from build123d import *

# Parameters (mm, degrees)
F1_DEPTH = 20


with BuildPart() as f1:
    # F0 (on Top) → F1 (new body)
    with BuildSketch(Plane.XY):
        with BuildLine():
            Line((-4.08337, 18.350895), (0, 18.350895))
            Line((0, 18.350895), (4.08337, 18.350895))
            ThreePointArc((4.08337, 18.350895), (8.797416, 19.531724), (12.398165, 22.795339))
            ThreePointArc((12.398165, 22.795339), (25.178356, 23.493196), (22.271844, 11.028346))
            ThreePointArc((22.271844, 11.028346), (18.432547, 8.049022), (16.451072, 3.611642))
            Line((16.451072, 3.611642), (12.878556, -16.649105))
            ThreePointArc((12.878556, -16.649105), (14.054737, -18.328866), (15.734498, -17.152685))
            Line((15.734498, -17.152685), (19.307015, 3.108062))
            ThreePointArc((19.307015, 3.108062), (20.713862, 6.258602), (23.439763, 8.373922))
            ThreePointArc((23.439763, 8.373922), (27.399884, 25.35728), (9.986874, 24.40645))
            ThreePointArc((9.986874, 24.40645), (7.430343, 22.089283), (4.08337, 21.250895))
            Line((4.08337, 21.250895), (0, 21.250895))
            Line((0, 21.250895), (-4.08337, 21.250895))
            ThreePointArc((-4.08337, 21.250895), (-7.430343, 22.089283), (-9.986874, 24.40645))
            ThreePointArc((-9.986874, 24.40645), (-27.399884, 25.35728), (-23.439763, 8.373922))
            ThreePointArc((-23.439763, 8.373922), (-20.713862, 6.258602), (-19.307015, 3.108062))
            Line((-19.307015, 3.108062), (-15.734498, -17.152685))
            ThreePointArc((-15.734498, -17.152685), (-14.054737, -18.328866), (-12.878556, -16.649105))
            Line((-12.878556, -16.649105), (-16.451072, 3.611642))
            ThreePointArc((-16.451072, 3.611642), (-18.432547, 8.049022), (-22.271844, 11.028346))
            ThreePointArc((-22.271844, 11.028346), (-25.178356, 23.493196), (-12.398165, 22.795339))
            ThreePointArc((-12.398165, 22.795339), (-8.797416, 19.531724), (-4.08337, 18.350895))
        make_face()
    extrude(amount=F1_DEPTH)


solid = f1.part
Build history of the part. All positions in model axes, mm. A direction names the side the tool comes from. Coordinates: 2 decimals unless noted, no trailing zeros. Order: outer loops, then holes, each group sorted by start corner. A loop starts at its lowest first (then second) coordinate and runs counter-clockwise, first axis right, second up. Notation, with made-up numbers: (-38, 72.25) - (-18, 72.25) arc R11 ccw to (-18, 91.25) - close; hole circle Ø9 at (63, -13). An arc over 180 degrees is marked (long way). Write each question's results on one line, items separated by ' | '. Start each with the question number.
Item 1: Band-saw the part on D-D on y = 7.5. Write the cut outline in (x, z).
Item 2: Band-saw the part on A-A on y = 23.5. Write the cut outline in (x, z), and give its area (3 significant figures).
Item 3: Band-saw the part on B-B on x = 26. Write the cut outline in (y, z), and give its area (3 significant figures).
Item 4: Tool access for faces 1 (the face through (-17.546, -6.88, 9.86)), 2 (the face through (0, 18.351, 10)), 3 (the face through (0, 21.251, 10)), 4 (the face through (-18.39, 7.995, 9.86)): list every direction of +Z, -Z, +X, -X, +Y, -Y with a clear straight run to the whole face (end or side of a thin tool).
Item 5: Flat gauge pins, fed straight in: pin 1 (6 mm diameter, centred on y = 7, z = 4.5, fed in from -X); pin 2 (2.5 mm diameter, centred on x = -1.5, z = 6.5, fed in from +Y); pin 3 (1 mm diameter, centred on x = 7, z = 10.5, fed in from +Y). Where does each tip first touch, or does it go through?
Item 6: Band-saw the part on C-C on z = 19. Write the cut outline in (x, y), and give its area (3 significant figures).
Item 7: Mould opens along X. For faces 5 (the face through (0, 20, 0)), 6 (the face through (-20.744, 6.297, 9.86)), 7 (the face through (20.684, 6.22, 9.86)), 8 (the face through (14.023, -18.323, 9.86)) say: released by +X, released by -X, zero draft, split by the parting line, or undercut.
Item 8: Wall check: probe 1 along X at (y, z) = (24, 19); probe 2 along Y at (x, z) = (-0.5, 14); probe 3 along X at (y, z) = (25, 11.75). Give the ranges that are in metal, low to high. Write a range as [from, to].
Numbers:
1) outline: (-21.97, 0) - (-18.03, 0) - (-18.03, 20) - (-21.97, 20) - close; (18.03, 0) - (21.97, 0) - (21.97, 20) - (18.03, 20) - close
2) outline: (-28.66, 0) - (-25.17, 0) - (-25.17, 20) - (-28.66, 20) - close; (-12.93, 0) - (-9.27, 0) - (-9.27, 20) - (-12.93, 20) - close; (9.27, 0) - (12.93, 0) - (12.93, 20) - (9.27, 20) - close; (25.17, 0) - (28.66, 0) - (28.66, 20) - (25.17, 20) - close | area: 286 mm^2
3) outline: (9.95, 0) - (14.39, 0) - (14.39, 20) - (9.95, 20) - close; (22.31, 0) - (26.75, 0) - (26.75, 20) - (22.31, 20) - close | area: 177 mm^2
4) face 1: +Z, -Z, -X, -Y | face 2: +Z, -Z, -Y | face 3: +Z, -Z, +Y | face 4: +Z, -Z
5) pin 1: x = -26.06 | pin 2: y = 21.25 | pin 3: y = 22.13
6) outline: (-23.44, 8.37) arc R7.1 cw to (-19.31, 3.11) - (-15.73, -17.15) arc R1.45 ccw to (-12.88, -16.65) - (-16.45, 3.61) arc R10 ccw to (-22.27, 11.03) arc R8 cw (long way) to (-12.4, 22.8) arc R10 ccw to (-4.08, 18.35) - (4.08, 18.35) arc R10 ccw to (12.4, 22.8) arc R8 cw (long way) to (22.27, 11.03) arc R10 ccw to (16.45, 3.61) - (12.88, -16.65) arc R1.45 ccw to (15.73, -17.15) - (19.31, 3.11) arc R7.1 cw to (23.44, 8.37) arc R10.9 ccw (long way) to (9.99, 24.41) arc R7.1 cw to (4.08, 21.25) - (-4.08, 21.25) arc R7.1 cw to (-9.99, 24.41) arc R10.9 ccw (long way) to start | area: 450 mm^2
7) face 5: zero draft | face 6: released by -X | face 7: released by +X | face 8: undercut
8) probe 1: [-28.37, -24.71], [-13.39, -9.69], [9.69, 13.39], [24.71, 28.37] | probe 2: [18.35, 21.25] | probe 3: [-27.69, -23.5], [-14.6, -10.41], [10.41, 14.6], [23.5, 27.69]
